Design review of the part built by this model. Coordinates are the model's own, in mm. A direction names the side the tool comes from. Give positions to 0.01 mm unless a question says otherwise; leave off trailing zeros. Write each loop counter-clockwise with the first axis right and the second up, starting at its lowest first coordinate (ties: lowest second). Pieces come first, ordered by that corner, then holes. Notation, with made-up numbers: M -28,49 L 14,49 A28 cw 14,82 Z; hole C -8,67 d4. An arc over 180 degrees is marked long. Use one line per item in the form item = value. Start each with the question number.
from build123d import *

# Parameters (mm, degrees)
SKETCH1_W           = 20
SKETCH1_H           = 10
BOSS_EXTRUDE1_DEPTH = 50
SKETCH2_R           = 3
CUT_EXTRUDE1_DEPTH  = 55.083269132
CUT_EXTRUDE2_DEPTH  = 14
LPATTERN1_COUNT     = 2
LPATTERN1_PITCH     = 41
FILLET1_DEPTH       = 50


with BuildPart() as part:
    # Sketch1 → Boss-Extrude1 (new body)
    with BuildSketch(Plane(origin=(0, 0, 0), x_dir=(1, 0, 0), z_dir=(0, 1, 0))):
        Rectangle(SKETCH1_W, SKETCH1_H)
    extrude(amount=BOSS_EXTRUDE1_DEPTH)

    # Sketch2 → Cut-Extrude1 (cut, through all)
    with BuildSketch(Plane(origin=(10, 0, 0), x_dir=(0, 0, -1), z_dir=(1, 0, 0))):
        with Locations((0, 4.509775146)):
            Circle(SKETCH2_R)
    cut_extrude1 = extrude(amount=-CUT_EXTRUDE1_DEPTH, mode=Mode.SUBTRACT)

    # Sketch3 → Cut-Extrude2 (cut)
    with BuildSketch(Plane(origin=(0, 0, -5), x_dir=(-1, 0, 0), z_dir=(0, 0, -1))):
        with BuildLine():
            Line((-4.941150344, 37.404706109), (-4.941150344, 42.795051939))
            ThreePointArc((-4.941150344, 42.795051939), (0, 47.736202283), (4.941150344, 42.795051939))
            Line((4.941150344, 42.795051939), (4.941150344, 37.404706109))
            ThreePointArc((4.941150344, 37.404706109), (0, 32.463555765), (-4.941150344, 37.404706109))
        make_face()
    extrude(amount=-CUT_EXTRUDE2_DEPTH, mode=Mode.SUBTRACT)

    # LPattern1: Cut-Extrude1 ×2
    with Locations(*[(0, i * LPATTERN1_PITCH, 0) for i in range(1, LPATTERN1_COUNT)]):
        add(cut_extrude1, mode=Mode.SUBTRACT)

    # Fillet1: read off the stored shape, not the designer's step
    # Fillet1 outline → Fillet1 (cut)
    with BuildSketch(Plane(origin=(0, 0, 0), x_dir=(1, 0, 0), z_dir=(0, 1, 0))):
        with BuildLine():
            ThreePointArc((0, 5), (7.071067812, 2.071067812), (10, -5))
            Line((10, -5), (10, 5))
            Line((10, 5), (0, 5))
        make_face()
        with BuildLine():
            Line((0, 5), (-10, 5))
            Line((-10, 5), (-10, -5))
            ThreePointArc((-10, -5), (-7.071067812, 2.071067812), (0, 5))
        make_face()
    extrude(amount=FILLET1_DEPTH, mode=Mode.SUBTRACT)


solid = part.part
1. We need section C-C (y = 3). State the section outline as (x, z) points, and give its area (3 significant figures).
2. We need section B-B (z = -2.5). State the section outline as (x, y) points, and give its area (3 significant figures).
3. We need section D-D (x = 9.25). State the section outline as (y, z) points, and give its area (3 significant figures).
4. We need section A-A (x = -1). State the section outline as (y, z) points.
5. Draft analysis for pull direction X (two halves, no side actions). For faces 1 (the flat face through (0, 50, 1)), 2 (the cylindrical face through (-0.109, 32.465, -0.07)), state which applies: pulls with the +X half, pulls with the -X half, needs draft (parallel to the pull), parting line crosses it, or undercut.
6. To check wall thickness, follow L1, parallel to Y at x = -4, z = 0; L2, parallel to Y at x = 3.5, z = 2.25; L3, parallel to Z at x = 1, y = 13.5. State the ranges of each line that lie inside material, in increasing order.
7. Clearance check with flat-ended pins moving along their axes: pin 1 Ø2.5 at (y, z) = (41, 0.5) entering from +X; pin 2 Ø1 at (y, z) = (20, -1.5) entering from -X; pin 3 Ø1.6 at (y, z) = (39.5, 0.5) entering from -X. State where each tip first meets the part, or that it passes through.
8. For faces 3 (the flat face through (4.941, 40, 1)), 4 (the flat face through (0, 0, 1)), list the 3-axis set-ups (+Z, -Z, +X, -X, +Y, -Y) from which the entire face can be reached by the end or side of a thin tool; tool diameter is ignored.
Answer block:
q1.outline = M -10,5 A10 ccw -9.71,2.59 L 9.71,2.59 A10 ccw 10,5 Z; M -6.51,-2.59 A10 ccw 6.51,-2.59 Z
q1.area = 69.1 mm^2
q2.outline = M -6.61,0 L 6.61,0 L 6.61,2.85 L -6.61,2.85 Z; M -6.61,6.17 L 6.61,6.17 L 6.61,43.85 L 4.83,43.85 A4.94 cw 4.94,42.8 L 4.94,37.4 A4.94 cw -4.94,37.4 L -4.94,42.8 A4.94 cw -4.83,43.85 L -6.61,43.85 Z; M -6.61,47.17 L -2.3,47.17 A4.94 cw 2.3,47.17 L 6.61,47.17 L 6.61,50 L -6.61,50 Z
q2.area = 470 mm^2
q3.outline = M 0,1.2 L 1.76,1.2 A3 cw 7.26,1.2 L 42.76,1.2 A3 cw 48.26,1.2 L 50,1.2 L 50,5 L 0,5 Z
q3.area = 176 mm^2
q4.outline = M 0,-4.95 L 32.57,-4.95 L 32.57,5 L 0,5 Z; M 47.63,-4.95 L 50,-4.95 L 50,5 L 47.63,5 L 47.63,2.12 A3 cw 47.63,-2.12 Z; hole C 4.51,0 d6
q5.face_1 = needs draft
q5.face_2 = undercut
q6.L1 = 0 to 1.51, 7.51 to 34.5, 48.51 to 50
q6.L2 = 0 to 2.53, 6.49 to 33.92, 47.49 to 50
q6.L3 = -4.95 to 5
q7.pin_1 = 9.46
q7.pin_2 = -8
q7.pin_3 = -9.29
q8.face_3 = +Z, -Z
q8.face_4 = +Z, -Z, +X, -X, -Y
